from build123d import *

# Parameters (mm, degrees)
F1_DEPTH = 38.1
F2_R     = 2.4892
F3_DEPTH = 50.801
F4_R     = 6.35
F5_DEPTH = 25.401


with BuildPart() as f1:
    # F0 (on Top) → F1 (new body)
    with BuildSketch(Plane.XY):
        Polygon((3.175, 50.8), (0, 50.8), (0, 0), (25.4, 0), (25.4, 3.175), (3.175, 3.175), align=None)
    extrude(amount=F1_DEPTH)

    # F2 (on face) → F3 (cut, through all)
    with BuildSketch(Plane.XZ):
        with Locations((12.7, 25.4)):
            Circle(F2_R)
        with Locations((12.7, 12.7)):
            Circle(F2_R)
    extrude(amount=-F3_DEPTH, mode=Mode.SUBTRACT)

    # F4 (on face) → F5 (cut, through all)
    with BuildSketch(Plane(origin=(0, 0, 0), x_dir=(0, -1, 0), z_dir=(-1, 0, 0))):
        with Locations((-38.1, 19.05)):
            Circle(F4_R)
    extrude(amount=-F5_DEPTH, mode=Mode.SUBTRACT)


solid = f1.part
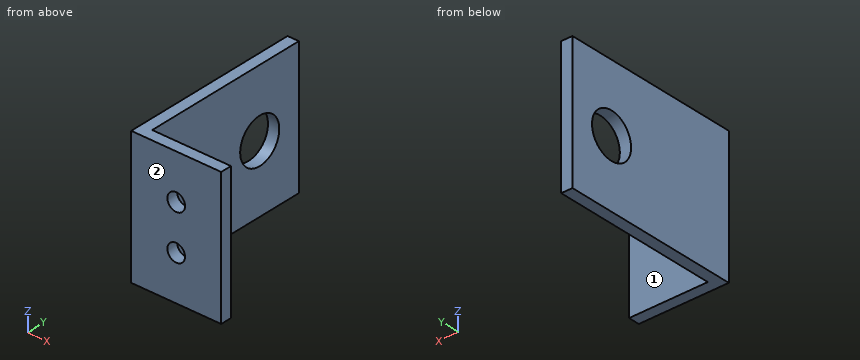
Build history of the part. All positions in model axes, mm. Face numbers are marked on the shaded views. A direction names the side the tool comes from. Coordinates: 2 decimals unless noted, no trailing zeros. Write each loop counter-clockwise with the first axis right and the second up, starting at its lowest first coordinate (ties: lowest second). Pieces come first, ordered by that corner, then holes.
(1) Pin check, flat tip, straight feed: pin 1 Ø19 at (y, z) = (22, 27.5) entering from +X (3 decimals). Stop position of the tip, or through.
(2) Drill centre lines: line 1 (Z direction, x = 12.7, y = 1.15); line 2 (Z direction, x = 2.3, y = 38.1); line 3 (Y direction, x = 14.5, z = 2.5) (3 decimals). Where is each one in solid material? Low to high.
(3) Cut at B-B on y = 38.1. List the corners of the cut face in (x, z) (3 decimals).
(4) Cut at C-C on z = 19.05. List the corners of the cut face in (x, y) (3 decimals).
(5) Cut at A-A on x = 12.7. List the corners of the cut face in (y, z) (3 decimals), and give its area (3 significant figures).
(6) 3-axis set-ups, long thin cutter, end or side, ignore diameter. For the marked faces 1 and 2: which of +Z, -Z, +X, -X, +Y, -Y reach the whole face in a straight line?
(7) Cut at D-D on z = 34. List the corners of the cut face in (x, y) (3 decimals), and give its area (3 significant figures).
Working result:
1. pin 1: stops at x = 3.175
2. line 1: z = 0 to 10.21, 15.19 to 22.91, 27.89 to 38.1
2. line 2: z = 0 to 12.7, 25.4 to 38.1
2. line 3: y = 0 to 3.175
3. outline: (0, 0) - (3.175, 0) - (3.175, 12.7) - (0, 12.7) - close; (0, 25.4) - (3.175, 25.4) - (3.175, 38.1) - (0, 38.1) - close
4. outline: (0, 0) - (25.4, 0) - (25.4, 3.175) - (3.175, 3.175) - (3.175, 31.75) - (0, 31.75) - close; (0, 44.45) - (3.175, 44.45) - (3.175, 50.8) - (0, 50.8) - close
5. outline: (0, 0) - (3.175, 0) - (3.175, 10.211) - (0, 10.211) - close; (0, 15.189) - (3.175, 15.189) - (3.175, 22.911) - (0, 22.911) - close; (0, 27.889) - (3.175, 27.889) - (3.175, 38.1) - (0, 38.1) - close
5. area: 89.4 mm2
6. face 1: +Z, -Z, +X, +Y
6. face 2: +Z, -Z, +X, -X, -Y
7. outline: (0, 0) - (25.4, 0) - (25.4, 3.175) - (3.175, 3.175) - (3.175, 50.8) - (0, 50.8) - close
7. area: 232 mm2
